Input: part model. Units: mm. Frame: model coordinates. A direction names the side the tool comes from. Give positions to 0.01 mm unless a question says otherwise; leave off trailing zeros. Loops run counter-clockwise (first coordinate to the right, second up) from the corner with the lowest first, then second, coordinate; pieces in that order, holes last. Notation, with made-up numbers: (44.5, -8.75) - (101.5, -8.75) arc R14 ccw to (101.5, 5.25) - close; hole circle Ø8 at (88.5, 17). An arc over 180 degrees is marked (long way). Answer as a JSON object with one key per item and string values.
Autodesk Inventor part; units mm, degrees
ref_plane "YZ Plane" through (0, 0, 0) normal (1, 0, 0) x (0, 1, 0)
ref_plane "XZ Plane" through (0, 0, 0) normal (0, 1, 0) x (-1, 0, 0)
ref_plane "XY Plane" through (0, 0, 0) normal (0, 0, 1) x (1, 0, 0)
sketch "Sketch1" plane through (0, 0, 0) normal (0, 1, 0) x (-1, 0, 0)
  circle A0 centre (0, 0) radius 2
  dimension "d0" = 4
extrude "Extrusion1" add sketch "Sketch1" along normal blind 1.5
sketch "Sketch2" plane through (0, 1.5, 0) normal (0, 1, 0) x (1, 0, 0)
  circle A0 centre (0, 0) radius 1.5
  dimension "d3" = 3
extrude "Extrusion2" add sketch "Sketch2" along normal blind 7
sketch "Sketch3" plane through (0, 0, 0) normal (0, -1, 0) x (1, 0, 0)
  line L0 (0.905, 0) -> (0.4525, -0.7838)
  line L1 (0.4525, -0.7838) -> (-0.4525, -0.7838)
  line L2 (-0.4525, -0.7838) -> (-0.905, 0)
  line L3 (-0.905, 0) -> (-0.4525, 0.7838)
  line L4 (-0.4525, 0.7838) -> (0.4525, 0.7838)
  line L5 (0.4525, 0.7838) -> (0.905, 0)
  point P0 (0, 0)
  point P1 (0, 0)
extrude "Extrusion3" cut sketch "Sketch3" against normal blind 1
fillet "Fillet1" radius 1 1 edges at (2, 0, 0)
thread "Thread1"
properties part number "M3x13"
Item 1: Mould query, pull axis X, two halves, no side actions, for faces 1 (the face through (0, 8.5, 0)), 2 (the face through (-1.5, 4.95, 0.07)), 3 (the face through (0, 1, 0)), 4 (the face through (0, 0.5, 0.784)). Classes: released by +X, released by -X, zero draft, split by the parting line, or undercut.
Geometry check:
{"face 1": "zero draft", "face 2": "split by the parting line", "face 3": "undercut", "face 4": "undercut"}
Item 2: Access query for faces 5 (the face through (0, 0.5, -0.784)), 6 (the face through (0.434, 1.246, 1.952)). Directions: +Z, -Z, +X, -X, +Y, -Y. A direction counts if a zero-diameter tool reaches every point of the face in a straight line with its end or side. Return the directions, or none.
Geometry check:
{"face 5": "-Y", "face 6": "+Y, -Y"}
Item 3: Cut plane A-A (y = 5). Return loops of the section in (x, z), then the cut area to 3 significant figures.
Geometry check:
{"outline": "circle Ø3 at (0, 0)", "area": "7.07 mm2"}
Item 4: Material intervals for line 1 (X direction, y = 5.5, z = 0.2); line 2 (Y direction, x = -0.85, z = -0.75); line 3 (Z direction, x = 1.15, y = 1), sorted ascending. Write a range as [from, to].
Geometry check:
{"line 1": "x = [-1.49, 1.49]", "line 2": "y = [0.01, 8.5]", "line 3": "z = [-1.64, 1.64]"}
Item 5: Contact query for flat-ended pins moving along their axis: P1, Ø0.7, axis at x = 0, y = 0.5, coming from the +Z side; P2, Ø0.5, axis at x = -0.5, z = 0, coming from the -Y side; P3, Ø1, axis at y = 3, z = 0, coming from the -X side. Output: stop coordinate, or through.
Geometry check:
{"P1": "stops at z = 1.99", "P2": "stops at y = 1", "P3": "stops at x = -1.5"}
